```python
from build123d import *

# Parameters (mm, degrees)
F0_R            = 63.5
F1_DEPTH        = 6.35
F2_DEPTH        = 12.7
F3_R            = 9.5319869965
F4_DEPTH        = 38.1
F4_COPIES_COUNT = 6


# Not quite as in the source:
# - a pattern or mirror of a feature is missing from the dataset's text; its kind, count and spacing are read off the source's solid


with BuildPart() as f1:
    # F0 (on Front) → F1 (new body)
    with BuildSketch(Plane.XZ):
        Circle(F0_R)
        with BuildLine():
            ThreePointArc((50.7040266498, 3.121166689), (50.7760009936, 1.5613209459), (50.8, 0))
            ThreePointArc((50.8, 0), (47.8083719104, -17.1755516731), (39.1858434932, -32.3281559902))
            Line((39.1858434932, -32.3281559902), (40.8804939154, -34.660642193))
            Line((40.8804939154, -34.660642193), (20.3314622583, -49.5903876012))
            Line((20.3314622583, -49.5903876012), (18.636811836, -47.2579013985))
            ThreePointArc((18.636811836, -47.2579013985), (0, -50.8), (-18.636811836, -47.2579013985))
            Line((-18.636811836, -47.2579013985), (-20.3314622583, -49.5903876012))
            Line((-20.3314622583, -49.5903876012), (-40.8804939154, -34.660642193))
            Line((-40.8804939154, -34.660642193), (-39.1858434932, -32.3281559902))
            ThreePointArc((-39.1858434932, -32.3281559902), (-48.3136710278, -15.6980633142), (-50.7040266498, 3.121166689))
            Line((-50.7040266498, 3.121166689), (-53.4460286321, 4.0120971402))
            Line((-53.4460286321, 4.0120971402), (-45.5969969749, 28.1689326541))
            Line((-45.5969969749, 28.1689326541), (-42.8549949926, 27.2780022029))
            ThreePointArc((-42.8549949926, 27.2780022029), (-29.8594908165, 41.0980633142), (-12.7, 49.1868884968))
            Line((-12.7, 49.1868884968), (-12.7, 52.07))
            Line((-12.7, 52.07), (12.7, 52.07))
            Line((12.7, 52.07), (12.7, 49.1868884968))
            ThreePointArc((12.7, 49.1868884968), (29.8594908165, 41.0980633142), (42.8549949926, 27.2780022029))
            Line((42.8549949926, 27.2780022029), (45.5969969749, 28.1689326541))
            Line((45.5969969749, 28.1689326541), (53.4460286321, 4.0120971402))
            Line((53.4460286321, 4.0120971402), (50.7040266498, 3.121166689))
        make_face(mode=Mode.SUBTRACT)
        with BuildLine():
            Line((-20.3314622583, -49.5903876012), (-18.636811836, -47.2579013985))
            ThreePointArc((-18.636811836, -47.2579013985), (-29.8594908165, -41.0980633142), (-39.1858434932, -32.3281559902))
            Line((-39.1858434932, -32.3281559902), (-40.8804939154, -34.660642193))
            Line((-40.8804939154, -34.660642193), (-20.3314622583, -49.5903876012))
        make_face()
        with BuildLine():
            ThreePointArc((-50.7040266498, 3.121166689), (-48.3136710278, 15.6980633142), (-42.8549949926, 27.2780022029))
            Line((-42.8549949926, 27.2780022029), (-45.5969969749, 28.1689326541))
            Line((-45.5969969749, 28.1689326541), (-53.4460286321, 4.0120971402))
            Line((-53.4460286321, 4.0120971402), (-50.7040266498, 3.121166689))
        make_face()
        with BuildLine():
            Line((40.8804939154, -34.660642193), (39.1858434932, -32.3281559902))
            ThreePointArc((39.1858434932, -32.3281559902), (29.8594908165, -41.0980633142), (18.636811836, -47.2579013985))
            Line((18.636811836, -47.2579013985), (20.3314622583, -49.5903876012))
            Line((20.3314622583, -49.5903876012), (40.8804939154, -34.660642193))
        make_face()
        with BuildLine():
            ThreePointArc((42.8549949926, 27.2780022029), (48.3136710278, 15.6980633142), (50.7040266498, 3.121166689))
            Line((50.7040266498, 3.121166689), (53.4460286321, 4.0120971402))
            Line((53.4460286321, 4.0120971402), (45.5969969749, 28.1689326541))
            Line((45.5969969749, 28.1689326541), (42.8549949926, 27.2780022029))
        make_face()
        with BuildLine():
            ThreePointArc((-12.7, 49.1868884968), (0, 50.8), (12.7, 49.1868884968))
            Line((12.7, 49.1868884968), (12.7, 52.07))
            Line((12.7, 52.07), (-12.7, 52.07))
            Line((-12.7, 52.07), (-12.7, 49.1868884968))
        make_face()
    extrude(amount=-F1_DEPTH)

    # F0 (on Front) → F2 (join)
    with BuildSketch(Plane.XZ):
        with BuildLine():
            ThreePointArc((39.1858434932, -32.3281559902), (47.8083719104, -17.1755516731), (50.8, 0))
            ThreePointArc((50.8, 0), (50.7760009936, 1.5613209459), (50.7040266498, 3.121166689))
            Line((50.7040266498, 3.121166689), (47.4068197536, 2.0498392259))
            Line((47.4068197536, 2.0498392259), (39.5577880965, 26.2066747398))
            Line((39.5577880965, 26.2066747398), (42.8549949926, 27.2780022029))
            ThreePointArc((42.8549949926, 27.2780022029), (29.8594908165, 41.0980633142), (12.7, 49.1868884968))
            Line((12.7, 49.1868884968), (12.7, 45.72))
            Line((12.7, 45.72), (-12.7, 45.72))
            Line((-12.7, 45.72), (-12.7, 49.1868884968))
            ThreePointArc((-12.7, 49.1868884968), (-29.8594908165, 41.0980633142), (-42.8549949926, 27.2780022029))
            Line((-42.8549949926, 27.2780022029), (-39.5577880965, 26.2066747398))
            Line((-39.5577880965, 26.2066747398), (-47.4068197536, 2.0498392259))
            Line((-47.4068197536, 2.0498392259), (-50.7040266498, 3.121166689))
            ThreePointArc((-50.7040266498, 3.121166689), (-48.3136710278, -15.6980633142), (-39.1858434932, -32.3281559902))
            Line((-39.1858434932, -32.3281559902), (-37.1480575634, -29.5233842787))
            Line((-37.1480575634, -29.5233842787), (-16.5990259063, -44.4531296869))
            Line((-16.5990259063, -44.4531296869), (-18.636811836, -47.2579013985))
            ThreePointArc((-18.636811836, -47.2579013985), (0, -50.8), (18.636811836, -47.2579013985))
            Line((18.636811836, -47.2579013985), (16.5990259063, -44.4531296869))
            Line((16.5990259063, -44.4531296869), (37.1480575634, -29.5233842787))
            Line((37.1480575634, -29.5233842787), (39.1858434932, -32.3281559902))
        make_face()
    extrude(amount=-F2_DEPTH)

    # F3 (on Front) → F4 (join)
    with BuildSketch(Plane.XZ):
        with Locations((51.6903102398, 0)):
            Circle(F3_R)
    f4 = extrude(amount=-F4_DEPTH)

    # F4_copies: F4 ×6 about axis
    f4_copies_axis = Axis((0, 0, 0), (0, 1, 0))
    for i in range(1, F4_COPIES_COUNT):
        add(f4.rotate(f4_copies_axis, i * 360 / F4_COPIES_COUNT))


solid = f1.part
```
Can you work these out from the model? Positions are in its coordinate system, mm. A direction names the side the tool comes from. Coordinates: 2 decimals unless noted, no trailing zeros. Loops run counter-clockwise (first coordinate to the right, second up) from the corner with the lowest first, then second, coordinate; pieces in that order, holes last.
Item 1: Suppose I cut it at A-A (x = 0). Please give me the cut outline in (y, z), then the cut area to 3 significant figures.
Answers below:
outline: (0, -63.5) - (6.35, -63.5) - (6.35, -50.8) - (12.7, -50.8) - (12.7, 45.72) - (0, 45.72) - close; (0, 50.8) - (6.35, 50.8) - (6.35, 63.5) - (0, 63.5) - close
area: 1,390 mm2
Item 2: I'm going to push flat-ended pins straight in: pin 1 (4 mm diameter, centred on x = 6, y = 5, fed in from -Z); pin 2 (3 mm diameter, centred on y = 8, z = 48, fed in from +X); pin 3 (3 mm diameter, centred on y = 4, z = 47, fed in from -X). Where does each tip first touch, or does it pass through?
Answers below:
pin 1: stops at z = -63.37
pin 2: stops at x = 35.22
pin 3: stops at x = -44.29
Item 3: Which directions (+Z, -Z, +X, -X, +Y, -Y) give clear straight access to the entire face, cutting with the end or side of a thin tool? Please do faces 1 (the face through (-1, 0, 0)), 2 (the face through (-32.87, 22, 51.21)), 3 (the face through (-32.98, 6.26, -32.55)).
Answers below:
face 1: +Z, -Z, +X, -X, -Y
face 2: +Y
face 3: +Y, -Y
Item 4: If we mould it in two halves opening along X, with no side actions, what happens to faces 4 (the face through (-26, 38.1, 45)), 5 (the face through (38.45, 9.48, 33.2)), 6 (the face through (36.31, 3.13, -35.53))? For each: released by +X, released by -X, zero draft, split by the parting line, or undercut.
Answers below:
face 4: zero draft
face 5: released by +X
face 6: undercut
Item 5: Suppose I cut it at D-D (z = 0). Please give me the cut outline in (x, y).
Answers below:
outline: (-63.5, 0) - (63.5, 0) - (63.5, 6.35) - (61.22, 6.35) - (61.22, 38.1) - (42.16, 38.1) - (42.16, 12.7) - (-42.16, 12.7) - (-42.16, 38.1) - (-61.22, 38.1) - (-61.22, 6.35) - (-63.5, 6.35) - close
Item 6: Please list where these lines run through material, in increasing order: L1, parallel to X at y = 2, z = -31; L2, parallel to X at y = 3, z = -33.5; L3, parallel to Z at x = -34.5, y = 7.5.
Answers below:
L1: x = -55.42 to -38.22, -35.12 to 35.12, 38.22 to 55.42
L2: x = -53.94 to -38.19, -31.67 to 31.67, 38.19 to 53.94
L3: z = -48.76 to -40.77, -31.45 to 37.29, 40.77 to 48.76
Item 7: Suppose I cut it at C-C (y = 30). Please give me the cut outline in (x, z), then the cut area to 3 significant figures.
Answers below:
outline: circle Ø19.06 at (-51.69, 0); circle Ø19.06 at (-25.85, -44.77); circle Ø19.06 at (-25.85, 44.77); circle Ø19.06 at (25.85, -44.77); circle Ø19.06 at (25.85, 44.77); circle Ø19.06 at (51.69, 0)
area: 1,710 mm2
Item 8: Suppose I cut it at B-B (y = 11). Please give me the cut outline in (x, z) (1 decimal).
Answers below:
outline: (-49.9, -9.4) arc R50.8 ccw to (-39.2, -32.3) - (-37.1, -29.5) - (-28.7, -35.7) arc R9.5 ccw (long way) to (-16.9, -47.9) arc R50.8 ccw to (16.9, -47.9) arc R9.5 ccw (long way) to (28.7, -35.7) - (37.1, -29.5) - (39.2, -32.3) arc R50.8 ccw to (49.9, -9.4) arc R9.5 ccw (long way) to (45.7, 7.4) - (39.6, 26.2) - (42.9, 27.3) arc R50.8 ccw to (33.1, 38.6) arc R9.5 ccw (long way) to (16.9, 47.9) arc R50.8 ccw to (12.7, 49.2) - (12.7, 45.7) - (-12.7, 45.7) - (-12.7, 49.2) arc R50.8 ccw to (-16.9, 47.9) arc R9.5 ccw (long way) to (-33.1, 38.6) arc R50.8 ccw to (-42.9, 27.3) - (-39.6, 26.2) - (-45.7, 7.4) arc R9.5 ccw (long way) to start
